Could you check a few things on this model? Use its own coordinates, in mm. A direction names the side the tool comes from. Round coordinates to 2 decimals unless told otherwise and drop trailing zeros. Write each loop counter-clockwise with the first axis right and the second up, starting at its lowest first coordinate (ties: lowest second). Pieces come first, ordered by that corner, then holes. Notation, with made-up numbers: (15, 50.25) - (58, 50.25) arc R14 cw to (58, 62.25) - close; hole circle Ø11 at (63, 1). An arc over 180 degrees is marked (long way). Write each question's results on one line, items separated by ' | '. Start each with the question number.
(1) Imagine slicing it at D-D on z = 34. Write out the boundary of the cut face in (x, y).
(2) Imagine slicing it at A-A on y = 15.5. Write out the boundary of the cut face in (x, z).
(3) Please list where these lines run through material, in increasing order: line 1 (Z direction, x = 213, y = -25.5); line 2 (Y direction, x = 50, z = 34); line 3 (Z direction, x = 254, y = 35). Write a range as [from, to].
(4) Thinking about a two-plate mould opening in Z: for faces 1 (the cylindrical face through (-260.599, -35.685, -2.736)), 2 (the cylindrical face through (4.27, 35.24, -48.08)), 3 (the flat face through (-304.8, -34, 0)), which applies, +Z half, -Z half, draft (parallel to the pull), parting line (faces both ways), or undercut?
(5) For P1, Ø8.5, axis at x = 254, z = 0, coming from the -Y side, with a flat end and sliding along its axis, tell me the tip position at first contact or that it passes through.
(6) Imagine slicing it at B-B on z = 0. State how many separate pieces and enclosed holes the cut face has, then the cut area to 3 significant figures.
(7) On a 3-axis mill with a long thin cutter (end or side, diameter ignored), from which of +Z, -Z, +X, -X, +Y, -Y can I reach the whole of each face in a straight line? I mean faces 4 (the flat face through (4, 0, 46.038)), 5 (the cylindrical face through (4.27, 35.38, 47.94)). Say none if no direction works.
```python
from build123d import *

# Parameters (mm, degrees)
F2_DEPTH = 304.8
F4_D     = 14.2875


# Not quite as in the source:
# - a variable given as a bare number and used for a length is read in inches; the dataset says mm whatever the document's units were


with BuildPart() as f2:
    # F1 (on Right) → F2 (new body, symmetric)
    with BuildSketch(Plane.YZ):
        with BuildLine():
            Line((28.575, 50.8), (-28.575, 50.8))
            ThreePointArc((-28.575, 50.8), (-35.3101920908, 48.0101920908), (-38.1, 41.275))
            Line((-38.1, 41.275), (-38.1, -41.275))
            ThreePointArc((-38.1, -41.275), (-35.3101920908, -48.0101920908), (-28.575, -50.8))
            Line((-28.575, -50.8), (28.575, -50.8))
            ThreePointArc((28.575, -50.8), (35.3101920908, -48.0101920908), (38.1, -41.275))
            Line((38.1, -41.275), (38.1, 41.275))
            ThreePointArc((38.1, 41.275), (35.3101920908, 48.0101920908), (28.575, 50.8))
        make_face()
        with BuildLine():
            ThreePointArc((-33.3375, 41.275), (-31.9425960454, 44.6425960454), (-28.575, 46.0375))
            Line((-28.575, 46.0375), (28.575, 46.0375))
            ThreePointArc((28.575, 46.0375), (31.9425960454, 44.6425960454), (33.3375, 41.275))
            Line((33.3375, 41.275), (33.3375, -41.275))
            ThreePointArc((33.3375, -41.275), (31.9425960454, -44.6425960454), (28.575, -46.0375))
            Line((28.575, -46.0375), (-28.575, -46.0375))
            ThreePointArc((-28.575, -46.0375), (-31.9425960454, -44.6425960454), (-33.3375, -41.275))
            Line((-33.3375, -41.275), (-33.3375, 41.275))
        make_face(mode=Mode.SUBTRACT)
    extrude(amount=F2_DEPTH, both=True)

    # F4 (through all)
    with Locations(Plane.XZ.offset(38.1)):
        with Locations((-254, 0), (0, 0), (254, 0)):
            Hole(F4_D / 2)


solid = f2.part
```
Response:
1) outline: (-304.8, -38.1) - (304.8, -38.1) - (304.8, -33.34) - (-304.8, -33.34) - close; (-304.8, 33.34) - (304.8, 33.34) - (304.8, 38.1) - (-304.8, 38.1) - close
2) outline: (-304.8, -50.8) - (304.8, -50.8) - (304.8, -46.04) - (-304.8, -46.04) - close; (-304.8, 46.04) - (304.8, 46.04) - (304.8, 50.8) - (-304.8, 50.8) - close
3) line 1: [-50.8, -46.04], [46.04, 50.8] | line 2: [-38.1, -33.34], [33.34, 38.1] | line 3: [-48.31, -7.14], [7.14, 48.31]
4) face 1: undercut | face 2: -Z half | face 3: draft
5) P1: through
6) separate pieces: 8 | enclosed holes: 0 | area: 5,400 mm²
7) face 4: +X, -X | face 5: +Z, +X, -X, +Y
